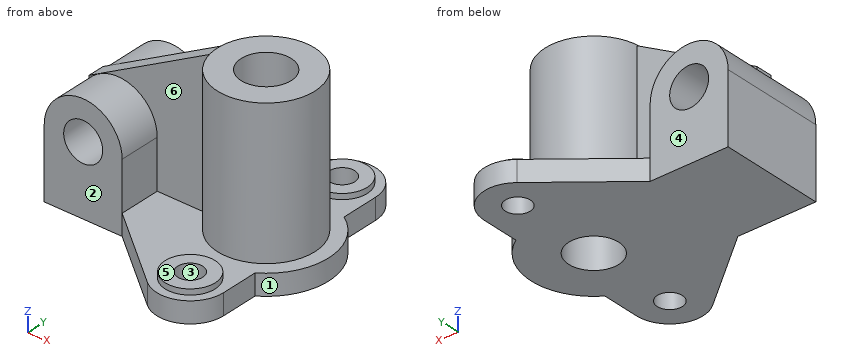
from build123d import *

# Parameters (mm, degrees)
F1_DEPTH  = 38.1
F0_W      = 142.24
F0_H      = 190.5
F2_DEPTH  = 127
F4_DEPTH  = 190.5
F5_R      = 35.56
F6_DEPTH  = 190.5
F7_R      = 45.72
F8_DEPTH  = 10.16
F9_DEPTH  = 10.16
F10_R     = 22.86
F11_DEPTH = 48.26
F12_R     = 22.86
F13_DEPTH = 48.26
F14_R     = 88.9
F15_DEPTH = 264.16
F16_R     = 45.72
F17_DEPTH = 302.26
F19_DEPTH = 30.48


with BuildPart() as f1:
    # F0 (on Top) → F1 (new body)
    with BuildSketch(Plane.XY):
        with BuildLine():
            Line((90.7176998631, 201.0186984875), (-53.7598490381, 83.8255537926))
            Line((-53.7598490381, 83.8255537926), (-53.7598490381, -106.6744462074))
            Line((-53.7598490381, -106.6744462074), (90.7176998631, -223.8675909024))
            ThreePointArc((90.7176998631, -223.8675909024), (155.3414036114, -231.5568685554), (190.0801509619, -176.5244462074))
            Line((190.0801509619, -176.5244462074), (190.0801509619, -108.1114070656))
            ThreePointArc((190.0801509619, -108.1114070656), (243.4201509619, -11.4244462074), (190.0801509619, 85.2625146508))
            Line((190.0801509619, 85.2625146508), (190.0801509619, 153.6755537926))
            ThreePointArc((190.0801509619, 153.6755537926), (155.3414036114, 208.7079761406), (90.7176998631, 201.0186984875))
        make_face()
    extrude(amount=F1_DEPTH)

    # F0 (on Top) → F2 (join)
    with BuildSketch(Plane.XY):
        with Locations((-124.8798490381, -11.4244462074)):
            Rectangle(F0_W, F0_H)
    extrude(amount=F2_DEPTH)

    # F3 (on face) → F4 (join)
    with BuildSketch(Plane.XZ.offset(106.6744462074)):
        with BuildLine():
            Line((-195.9998490381, 127), (-53.7598490381, 127))
            ThreePointArc((-53.7598490381, 127), (-124.8798490381, 198.12), (-195.9998490381, 127))
        make_face()
    extrude(amount=-F4_DEPTH)

    # F5 (on face) → F6 (cut)
    with BuildSketch(Plane.XZ.offset(106.6744462074)):
        with Locations((-124.8798490381, 127)):
            Circle(F5_R)
    extrude(amount=-F6_DEPTH, mode=Mode.SUBTRACT)

    # F7 (on face) → F8 (join)
    with BuildSketch(Plane.XY.offset(38.1)):
        with Locations((129.1201509619, -176.5244462074)):
            Circle(F7_R)
    extrude(amount=F8_DEPTH)

    # F7 (on face) → F9 (join)
    with BuildSketch(Plane.XY.offset(38.1)):
        with Locations((129.1201509619, 153.6755537926)):
            Circle(F7_R)
        with Locations((129.1201509619, -176.5244462074)):
            Circle(F7_R)
    extrude(amount=F9_DEPTH)

    # F10 (on face) → F11 (cut)
    with BuildSketch(Plane.XY.offset(48.26)):
        with Locations((129.1201509619, 153.6755537926)):
            Circle(F10_R)
    extrude(amount=-F11_DEPTH, mode=Mode.SUBTRACT)

    # F12 (on face) → F13 (cut)
    with BuildSketch(Plane.XY.offset(48.26)):
        with Locations((129.1201509619, -176.5244462074)):
            Circle(F12_R)
    extrude(amount=-F13_DEPTH, mode=Mode.SUBTRACT)

    # F14 (on face) → F15 (join)
    with BuildSketch(Plane.XY.offset(38.1)):
        with Locations((129.1201509619, -11.4244462074)):
            Circle(F14_R)
    extrude(amount=F15_DEPTH)

    # F16 (on face) → F17 (cut)
    with BuildSketch(Plane.XY.offset(302.26)):
        with Locations((129.1201509619, -11.4244462074)):
            Circle(F16_R)
    extrude(amount=-F17_DEPTH, mode=Mode.SUBTRACT)

    # F18 (on Front) → F19 (join)
    with BuildSketch(Plane.XZ):
        Polygon((43.5996614397, 302.26), (-178.0664920807, 179.1791468859), (-178.0664920807, 0), (43.5996614397, 0), align=None)
    extrude(amount=F19_DEPTH)


solid = f1.part
CAD build for the part. Positions are in the model's coordinates, mm. Face numbers are marked on the shaded views. A direction names the side the tool comes from. Coordinates: 2 decimals unless noted, no trailing zeros. Order: outer loops, then holes, each group sorted by start corner. A loop starts at its lowest first (then second) coordinate and runs counter-clockwise, first axis right, second up.
Item 1: 3-axis set-ups, long thin cutter, end or side, ignore diameter. For the marked faces 4, 5 and 6: which of +Z, -Z, +X, -X, +Y, -Y reach the whole face in a straight line?
Check sheet entries:
face 4: +Z, -Z, -X, +Y
face 5: +Z, +X, -X, -Y
face 6: +Z, -Y
Item 2: Band-saw the part on B-B on x = 98.5. List the corners of the cut face in (y, z).
Check sheet entries:
outline: (-229.24, 0) - (-45.38, 0) - (-45.38, 302.26) - (-94.88, 302.26) - (-94.88, 38.1) - (-142.57, 38.1) - (-142.57, 48.26) - (-210.48, 48.26) - (-210.48, 38.1) - (-229.24, 38.1) - close; (22.53, 0) - (206.39, 0) - (206.39, 38.1) - (187.63, 38.1) - (187.63, 48.26) - (119.72, 48.26) - (119.72, 38.1) - (72.04, 38.1) - (72.04, 302.26) - (22.53, 302.26) - close
Item 3: Pin check, flat tips, straight feed: pin 1 Ø19 at (y, z) = (112, 28) entering from +X; pin 2 Ø21.5 at (x, z) = (-128.5, 133) entering from +Y; pin 3 Ø12 at (x, z) = (-36, 223) entering from -Y. Stop position of each tip, or through.
Check sheet entries:
pin 1: stops at x = 190.08
pin 2: stops at y = 0
pin 3: stops at y = -30.48
Item 4: Drill centre lines: L1, parallel to Y at x = 112, z = 215; L2, parallel to Y at x = 145.5, z = 157; L3, parallel to Y at x = -144.5, z = 174. Where is each one in solid material? Low to high.
Check sheet entries:
L1: y = -98.66 to -53.82, 30.97 to 75.81
L2: y = -98.8 to -54.11, 31.26 to 75.95
L3: y = -106.67 to 83.83
Item 5: Band-saw the part on A-A on y = -39.5. List the corners of the cut face in (x, z), plus the area to 3 significant figures.
Check sheet entries:
outline: (-196, 0) - (93.04, 0) - (93.04, 302.26) - (44.77, 302.26) - (44.77, 38.1) - (-53.76, 38.1) - (-53.76, 127) arc R71.12 ccw to (-196, 127) - close; (165.2, 0) - (239.92, 0) - (239.92, 38.1) - (213.47, 38.1) - (213.47, 302.26) - (165.2, 302.26) - close; hole circle Ø71.12 at (-124.88, 127)
area: 56,000 mm2
Item 6: Band-saw the part on C-C on z = 207. List the corners of the cut face in (x, y).
Check sheet entries:
outline: (-127.96, -30.48) - (42.29, -30.48) arc R88.9 ccw (long way) to (40.96, 0) - (-127.96, 0) - close; hole circle Ø91.44 at (129.12, -11.42)
Item 7: Two-plate mould, pull along Y, no slides. Class the marked faces 1, 2 and 3: +Y half, -Y half, draft (parallel to the pull), parting line (faces both ways), or undercut.
Check sheet entries:
face 1: parting line
face 2: -Y half
face 3: undercut
Item 8: Band-saw the part on D-D on x = 3. List the corners of the cut face in (y, z), plus the area to 3 significant figures.
Check sheet entries:
outline: (-152.72, 0) - (129.87, 0) - (129.87, 38.1) - (0, 38.1) - (0, 279.72) - (-30.48, 279.72) - (-30.48, 38.1) - (-152.72, 38.1) - close
area: 18,100 mm2
